Part print with two shaded views. Sizes in mm from the minimum x, y, z corner. A direction names the side the tool comes from. Round coordinates to 2 decimals unless told otherwise and drop trailing zeros. Loops run counter-clockwise (first coordinate to the right, second up) from the corner with the lowest first, then second, coordinate; pieces in that order, holes last.
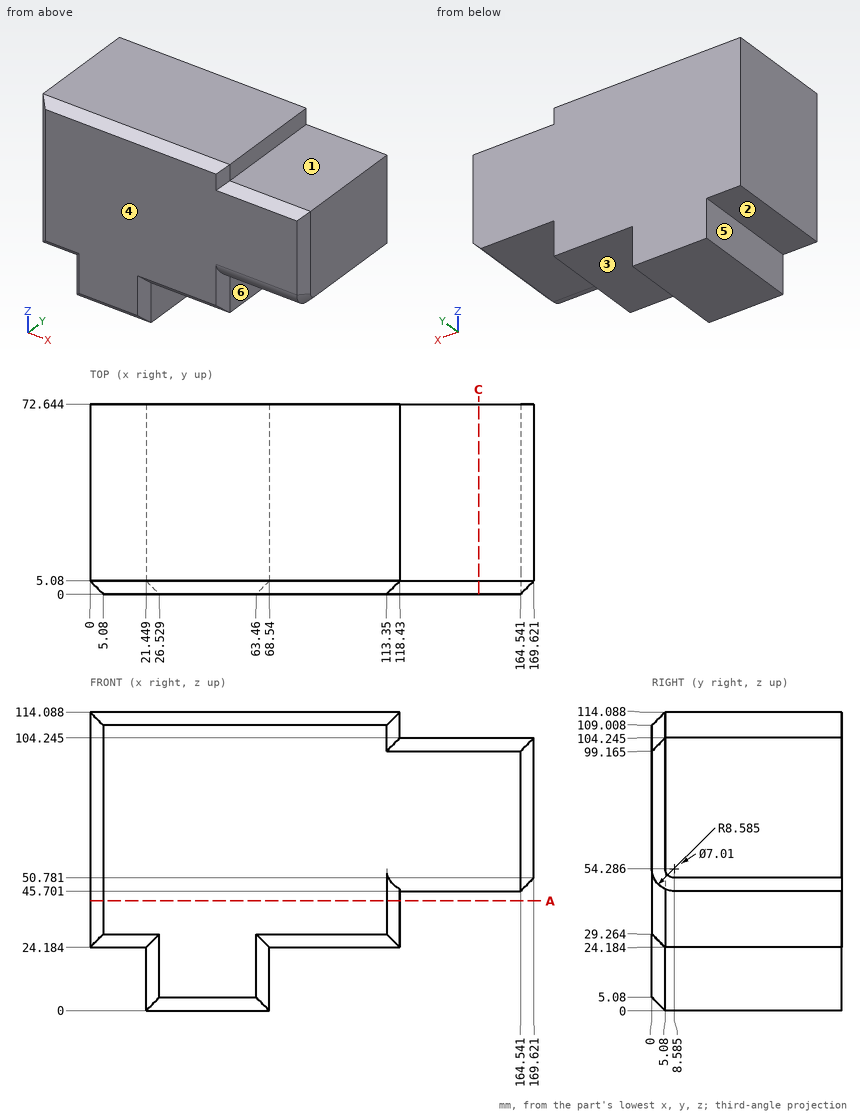
Item 1: Cut at C-C (x = 148.5). List the corners of the cut face in (y, z) (1 decimal).
Verdict:
outline: (0, 54.3) arc R8.6 ccw to (8.6, 45.7) - (72.6, 45.7) - (72.6, 104.2) - (5.1, 104.2) - (0, 99.2) - close
Item 2: Wall check: L1, parallel to Z at x = 157, y = 14.5 (1 decimal); L2, parallel to Z at x = 16, y = 55 (1 decimal); L3, parallel to X at y = 18.5, z = 29. Give the ranges that are in metal, low to high.
Verdict:
L1: z = 45.7 to 104.2
L2: z = 24.2 to 114.1
L3: x = 0 to 118.43
Item 3: Flat gauge pins, fed straight in: P1, Ø18, axis at y = 30.5, z = 39.5, coming from the +X side; P2, Ø4, axis at y = 44, z = 18.5, coming from the -X side; P3, Ø23.5, axis at x = 6, y = 33, coming from the -Z side (1 decimal). Where does each tip first touch, or does it go through?
Verdict:
P1: stops at x = 167.34
P2: stops at x = 21.45
P3: stops at z = 24.2
Item 4: Mould opens along X. For the marked faces 4, 5 and 6 say: released by +X, released by -X, zero draft, split by the parting line, or undercut.
Verdict:
face 4: zero draft
face 5: released by -X
face 6: released by +X
Item 5: 3-axis set-ups, long thin cutter, end or side, ignore diameter. For the marked faces 1, 2 and 3: which of +Z, -Z, +X, -X, +Y, -Y reach the whole face in a straight line?
Verdict:
face 1: +Z, +X, +Y, -Y
face 2: -Z, -X, +Y, -Y
face 3: -Z, +X, +Y, -Y
Item 6: Cut at A-A (z = 42). List the corners of the cut face in (x, y), plus the area to 3 significant figures.
Verdict:
outline: (0, 5.08) - (5.08, 0) - (113.35, 0) - (118.43, 5.08) - (118.43, 72.64) - (0, 72.64) - close
area: 8,580 mm2
